The model under review builds one solid part; all positions refer to its coordinate system, in mm. Face numbers are marked on the shaded views. A direction names the side the tool comes from. Round coordinates to 2 decimals unless told otherwise and drop trailing zeros.
1) Machinability: for the marked faces 1, 2 and 3, which of the approach directions +Z, -Z, +X, -X, +Y, -Y give a long, thin tool a straight path to every point of the face, cutting with its end or side? Answer none if there is none.
2) Mouldability with a two-part tool opening along X and no side actions: class the marked faces 4, 5 and 6 as pulls with the +X half, pulls with the -X half, needs draft (parallel to the pull), parting line crosses it, or undercut.
3) To check wall thickness, follow L1, parallel to X at y = 52, z = -3.5; L2, parallel to Y at x = 12, z = -41.5; L3, parallel to Y at x = 51.5, z = -43.5. State the ranges of each line that lie inside material, in increasing order.
4) Clearance check with flat-ended pins moving along their axes: P1, Ø2, axis at x = -5.5, z = -35.5, coming from the -Y side; P2, Ø12, axis at y = 67.5, z = -34.5, coming from the -X side; P3, Ø14, axis at x = -35, z = -50.5, coming from the +Y side; P4, Ø6, axis at y = 67, z = -67.5, coming from the -X side. State where each tip first meets the part, or that it passes through.
5) Consider section A-A (z = -43.5). Give the number of separate pieces and of enclosed holes in the cut face, then the cut area to 3 significant figures.
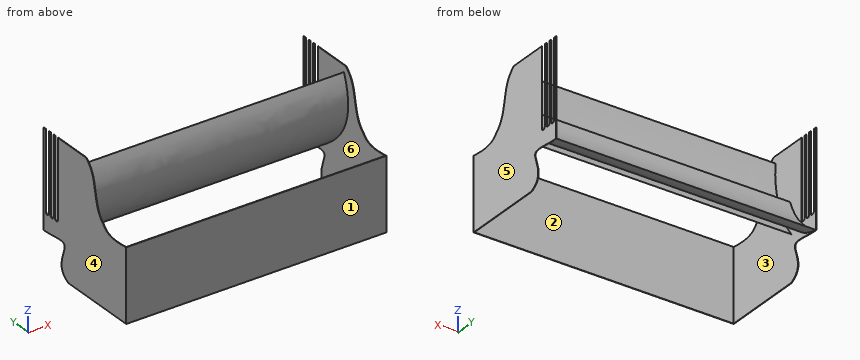
from build123d import *

# Parameters (mm, degrees)
BOSS_EXTRUDE1_START        = 762
BOSS_EXTRUDE1_DEPTH        = 2.54
BOSS_EXTRUDE3_DEPTH        = 759.46
BOSS_EXTRUDE3_DEPTH_BACK   = 762
BOSS_EXTRUDE3_2_DEPTH      = 759.46
BOSS_EXTRUDE3_2_DEPTH_BACK = 762
SKETCH13_W                 = 1524
SKETCH13_H                 = 423.429853573
BOSS_EXTRUDE4_DEPTH        = 2.54
CUT_EXTRUDE1_DEPTH         = 1278.344761778
CUT_EXTRUDE1_DEPTH_BACK    = 1278.344761778
CUT_EXTRUDE2_DEPTH         = 1278.344761778
CUT_EXTRUDE2_DEPTH_BACK    = 1278.344761778
SCALE1_SCALE               = 0.11


with BuildPart() as part:
    # Sketch3 → Boss-Extrude1 (new body)
    with BuildSketch(Plane(origin=(0, 0, 0), x_dir=(0, 0, -1), z_dir=(1, 0, 0)).offset(BOSS_EXTRUDE1_START)):
        with BuildLine():
            Line((338.570146427, 0), (762, 0))
            Line((762, 0), (762, 478.643823899))
            add(Edge.make_bspline(
                [(566.02119263, 685.8), (566.02119263, 609.562833411), (511.018643959, 418.064816879), (711.566045078, 596.214023542), (762, 478.643823899)],
                knots=[0, 0, 0, 0, 0.43337684, 1, 1, 1, 1], degree=3))
            Line((566.02119263, 685.8), (0, 685.8))
            Line((0, 685.8), (0, 216.97447871))
            add(Edge.make_bspline(
                [(0, 216.97447871), (268.153594246, 216.97447871), (370.795901917, 243.07894269), (338.570146427, 0)],
                knots=[0, 0, 0, 0, 1, 1, 1, 1], degree=3))
        make_face()
    extrude(amount=-BOSS_EXTRUDE1_DEPTH)


with BuildPart() as body_2:
    # Mirror1: mirrored copy
    add(part.part.mirror(Plane(origin=(0, 0, 0), x_dir=(0, 0, 1), z_dir=(1, 0, 0))))


with BuildPart() as body_3:
    # Sketch8 → Boss-Extrude3 (new, two sides: drawn at the far end of the back side and taken through both)
    with BuildSketch(Plane(origin=(0, 0, 0), x_dir=(0, 0, -1), z_dir=(1, 0, 0)).offset(-BOSS_EXTRUDE3_DEPTH_BACK)):
        with BuildLine():
            add(Edge.make_bspline(
                [(566.02119263, 685.8), (478.94605907, 530.59259106), (310.041791286, 470.260887435)],
                knots=[0, 0, 0, 1, 1, 1], degree=2))
            add(Edge.make_bspline(
                [(566.02119263, 685.8), (535.192963113, 473.791997419), (310.041791286, 470.260887435)],
                knots=[0, 0, 0, 1, 1, 1], degree=2))
        make_face()
    extrude(amount=BOSS_EXTRUDE3_DEPTH + BOSS_EXTRUDE3_DEPTH_BACK)


with BuildPart() as body_4:
    # Sketch8 → Boss-Extrude3 2 (new, two sides: drawn at the far end of the back side and taken through both)
    with BuildSketch(Plane(origin=(0, 0, 0), x_dir=(0, 0, -1), z_dir=(1, 0, 0)).offset(-BOSS_EXTRUDE3_2_DEPTH_BACK)):
        with BuildLine():
            add(Edge.make_bspline(
                [(493.805357443, 481.17753493), (291.820165627, 335.217986135), (39.854765798, 348.358323747)],
                knots=[0, 0, 0, 1, 1, 1], degree=2))
            add(Edge.make_bspline(
                [(493.805357443, 481.17753493), (323.598432885, 237.863082713), (39.854765798, 348.358323747)],
                knots=[0, 0, 0, 1, 1, 1], degree=2))
        make_face()
    extrude(amount=BOSS_EXTRUDE3_2_DEPTH + BOSS_EXTRUDE3_2_DEPTH_BACK)


with BuildPart() as part_1:
    add(part.part)

    add(body_2.part)  # Boss-Extrude4 merges body 2
    # Sketch13 → Boss-Extrude4 (add)
    with BuildSketch(Plane(origin=(0, 0, 0), x_dir=(1, 0, 0), z_dir=(0, 1, 0))):
        with Locations((0, 550.285073214)):
            Rectangle(SKETCH13_W, SKETCH13_H)
    extrude(amount=BOSS_EXTRUDE4_DEPTH)

    # Sketch16 → Cut-Extrude1 (cut, two sides: drawn at the far end of the back side and taken through both)
    with BuildSketch(Plane(origin=(0, 0, 0), x_dir=(0, 0, -1), z_dir=(1, 0, 0)).offset(-CUT_EXTRUDE1_DEPTH_BACK)):
        with BuildLine():
            Line((0, 667.670249742), (454.687424311, 667.670249742))
            ThreePointArc((454.687424311, 667.670249742), (467.387424311, 654.970249742), (454.687424311, 642.270249742))
            Line((454.687424311, 642.270249742), (0, 642.270249742))
            ThreePointArc((0, 642.270249742), (-12.7, 654.970249742), (0, 667.670249742))
        make_face()
        with BuildLine():
            Line((0, 604.170249742), (454.687424311, 604.170249742))
            ThreePointArc((454.687424311, 604.170249742), (467.387424311, 616.870249742), (454.687424311, 629.570249742))
            Line((454.687424311, 629.570249742), (0, 629.570249742))
            ThreePointArc((0, 629.570249742), (-12.7, 616.870249742), (0, 604.170249742))
        make_face()
        with BuildLine():
            Line((0, 566.070249742), (454.687424311, 566.070249742))
            ThreePointArc((454.687424311, 566.070249742), (467.387424311, 578.770249742), (454.687424311, 591.470249742))
            Line((454.687424311, 591.470249742), (0, 591.470249742))
            ThreePointArc((0, 591.470249742), (-12.7, 578.770249742), (0, 566.070249742))
        make_face()
    extrude(amount=CUT_EXTRUDE1_DEPTH + CUT_EXTRUDE1_DEPTH_BACK, mode=Mode.SUBTRACT)

    # Sketch17 → Cut-Extrude2 (cut, two sides: drawn at the far end of the back side and taken through both)
    with BuildSketch(Plane(origin=(0, 0, 0), x_dir=(0, 0, -1), z_dir=(1, 0, 0)).offset(-CUT_EXTRUDE2_DEPTH_BACK)):
        with BuildLine():
            Line((0, 334.71225841), (0, 103.643051311))
            Line((0, 103.643051311), (302.999558796, 187.654799067))
            add(Edge.make_bspline(
                [(302.999558796, 187.654799067), (225.21849282, 285.739628908), (76.800772912, 227.85117527), (0, 334.71225841)],
                knots=[0, 0, 0, 0, 1, 1, 1, 1], degree=3))
        make_face()
    extrude(amount=CUT_EXTRUDE2_DEPTH + CUT_EXTRUDE2_DEPTH_BACK, mode=Mode.SUBTRACT)

    # Combine1: union body 4, body 3
    add(body_4.part)
    add(body_3.part)


with BuildPart() as part_2:
    # Scale1: scaled about (0, 0, 0)
    add(part_1.part.scale(SCALE1_SCALE))


solid = part_2.part
Answer below:
1. face 1: +Z, -Z, +X, -X, -Y
1. face 2: +Z, -Z
1. face 3: none
2. face 4: pulls with the -X half
2. face 5: pulls with the +X half
2. face 6: undercut
3. L1: x = -83.82 to -83.54, 83.54 to 83.82
3. L2: y = 0 to 0.28, 40.07 to 45.34, 52.44 to 54.97
3. L3: y = 0 to 0.28, 41.46 to 46.31, 52.89 to 56.08
4. P1: stops at y = 36.56
4. P2: stops at x = -83.82
4. P3: stops at y = 68.29
4. P4: passes through
5. separate pieces: 7
5. enclosed holes: 2
5. area: 1,430 mm2
